```python
from build123d import *

# Parameters (mm, degrees)
SKETCH1_W               = 54
SKETCH1_H               = 32
SKETCH1_R               = 0.95
BOSS_EXTRUDE1_DEPTH     = 2.54
SKETCH3_W               = 3
SKETCH3_H               = 32
BOSS_EXTRUDE2_DEPTH     = 37
SKETCH4_W               = 32
SKETCH4_H               = 3
BOSS_EXTRUDE3_DEPTH     = 47
FILLET1_R               = 2
SKETCH5_R               = 1.425
CUT_EXTRUDE1_DEPTH      = 20
SKETCH8_W               = 32
SKETCH8_H               = 3
BOSS_EXTRUDE4_DEPTH     = 4
SKETCH7_W               = 5
SKETCH7_H               = 26
CUT_EXTRUDE3_DEPTH      = 1
CUT_EXTRUDE3_DEPTH_BACK = 40.54
CHAMFER1_SIZE           = 1.5


with BuildPart() as part:
    # Sketch1 → Boss-Extrude1 (new body)
    with BuildSketch(Plane(origin=(0, 0, 0), x_dir=(1, 0, 0), z_dir=(0, 1, 0))):
        with Locations((1, -10)):
            Rectangle(SKETCH1_W, SKETCH1_H)
        with Locations((-10, 0)):
            Circle(SKETCH1_R, mode=Mode.SUBTRACT)
        with Locations((20, -10)):
            Circle(SKETCH1_R, mode=Mode.SUBTRACT)
        with Locations((-10, -20)):
            Circle(SKETCH1_R, mode=Mode.SUBTRACT)
    extrude(amount=BOSS_EXTRUDE1_DEPTH)

    # Sketch3 → Boss-Extrude2 (add)
    with BuildSketch(Plane(origin=(0, 2.54, 0), x_dir=(1, 0, 0), z_dir=(0, 1, 0))):
        with Locations((26.5, -10)):
            Rectangle(SKETCH3_W, SKETCH3_H)
    extrude(amount=BOSS_EXTRUDE2_DEPTH)

    # Sketch4 → Boss-Extrude3 (add)
    with BuildSketch(Plane.ZY.offset(-25)):
        with Locations((10, 38.04)):
            Rectangle(SKETCH4_W, SKETCH4_H)
    extrude(amount=BOSS_EXTRUDE3_DEPTH)

    # Fillet1
    fillet1_edges = [part.edges().sort_by_distance(p)[0] for p in [
        (28, 0, 10),
        (28, 39.54, 10),
    ]]
    fillet(fillet1_edges, radius=FILLET1_R)

    # Sketch5 → Cut-Extrude1 (cut)
    with BuildSketch(Plane(origin=(0, 39.54, 0), x_dir=(1, 0, 0), z_dir=(0, 1, 0))):
        with Locations((-9.5, 2.5)):
            Circle(SKETCH5_R)
        with Locations((15.5, 2.5)):
            Circle(SKETCH5_R)
        with Locations((15.5, -22.5)):
            Circle(SKETCH5_R)
        with Locations((-9.5, -22.5)):
            Circle(SKETCH5_R)
    extrude(amount=-CUT_EXTRUDE1_DEPTH, mode=Mode.SUBTRACT)

    # Sketch8 → Boss-Extrude4 (add)
    with BuildSketch(Plane.ZY.offset(22)):
        with Locations((10, 38.04)):
            Rectangle(SKETCH8_W, SKETCH8_H)
    extrude(amount=BOSS_EXTRUDE4_DEPTH)

    # Sketch7 → Cut-Extrude3 (cut, two sides)
    with BuildSketch(Plane(origin=(0, 39.54, 0), x_dir=(1, 0, 0), z_dir=(0, 1, 0))) as cut_extrude3_sk:
        with Locations((-21.5, -10)):
            Rectangle(SKETCH7_W, SKETCH7_H)
    extrude(amount=CUT_EXTRUDE3_DEPTH, mode=Mode.SUBTRACT)
    extrude(cut_extrude3_sk.sketch, amount=-CUT_EXTRUDE3_DEPTH_BACK, mode=Mode.SUBTRACT)

    # Chamfer1
    chamfer1_edges = [part.edges().sort_by_distance(p)[0] for p in [
        (25, 2.54, 10),
        (25, 36.54, 10),
    ]]
    chamfer(chamfer1_edges, length=CHAMFER1_SIZE)


solid = part.part
```
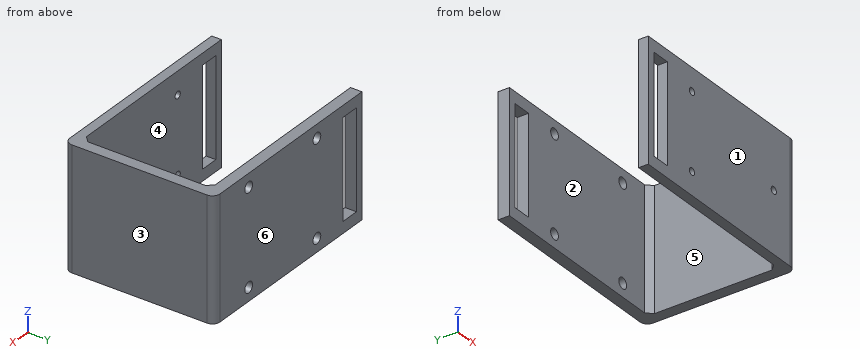
Source: CAD feature listing. Evaluate the final solid. Frame: model axes, mm. Face numbers are marked on the shaded views. A direction names the side the tool comes from. Give positions to 0.01 mm unless a question says otherwise; leave off trailing zeros. Write each loop counter-clockwise with the first axis right and the second up, starting at its lowest first coordinate (ties: lowest second). Pieces come first, ordered by that corner, then holes.
1. Section query D-D (z = 0). Return the cut outline in (x, y), then the cut area to 3 significant figures.
2. First-contact query: pin 1 (5 mm diameter, centred on y = 14.5, z = 1.5, fed in from -X); pin 2 (2.5 mm diameter, centred on x = 15.5, z = -2.5, fed in from +Y); pin 3 (1.1 mm diameter, centred on x = -10, z = 20, fed in from -Y). Flat tips, straight axial feed; report the tip coordinate or a pass-through.
3. Access query for the marked faces 1 and 2. Directions: +Z, -Z, +X, -X, +Y, -Y. A direction counts if a zero-diameter tool reaches every point of the face in a straight line with its end or side. Return the directions, or none.
4. Section query A-A (x = 22). Return the cut outline in (y, z).
5. Section query B-B (x = 15.5). Return the cut outline in (y, z) (3 decimals).
6. Pull-direction query (Y, two-part tool) for the marked faces 3, 4, 5 and 6; classes: +Y half, -Y half, draft (parallel to the pull), parting line (faces both ways), or undercut.
7. Material intervals for line 1 along Z through (x, y) = (-9.5, 37.7) (3 decimals); line 2 along Z through (x, y) = (-10, 1.3); line 3 along Y through (x, z) = (2.5, 3.5), sorted ascending.
8. Section query C-C (z = 17). Return the cut outline in (x, y), then the cut area to 3 significant figures.
Output values:
1. outline: (-26, 0) - (-24, 0) - (-24, 2.54) - (-26, 2.54) - close; (-26, 36.54) - (-24, 36.54) - (-24, 39.54) - (-26, 39.54) - close; (-19, 0) - (-10.95, 0) - (-10.95, 2.54) - (-19, 2.54) - close; (-19, 36.54) - (23.5, 36.54) - (25, 35.04) - (25, 4.04) - (23.5, 2.54) - (-9.05, 2.54) - (-9.05, 0) - (26, 0) arc R2 ccw to (28, 2) - (28, 37.54) arc R2 ccw to (26, 39.54) - (-19, 39.54) - close
1. area: 369 mm2
2. pin 1: stops at x = 25
2. pin 2: stops at y = 2.54
2. pin 3: stops at y = 36.54
3. face 1: +Z, -Z, +X, -X, -Y
3. face 2: +Z, -Z, -X
4. outline: (0, -6) - (2.54, -6) - (2.54, 26) - (0, 26) - close; (36.54, -6) - (39.54, -6) - (39.54, 26) - (36.54, 26) - close
5. outline: (0, -6) - (2.54, -6) - (2.54, 26) - (0, 26) - close; (36.54, -6) - (39.54, -6) - (39.54, -3.925) - (36.54, -3.925) - close; (36.54, -1.075) - (39.54, -1.075) - (39.54, 21.075) - (36.54, 21.075) - close; (36.54, 23.925) - (39.54, 23.925) - (39.54, 26) - (36.54, 26) - close
6. face 3: draft
6. face 4: undercut
6. face 5: undercut
6. face 6: +Y half
7. line 1: z = -6 to -3.925, -1.075 to 21.075, 23.925 to 26
7. line 2: z = -6 to -0.95, 0.95 to 19.05, 20.95 to 26
7. line 3: y = 0 to 2.54, 36.54 to 39.54
8. outline: (-26, 0) - (-24, 0) - (-24, 2.54) - (-26, 2.54) - close; (-26, 36.54) - (-24, 36.54) - (-24, 39.54) - (-26, 39.54) - close; (-19, 0) - (26, 0) arc R2 ccw to (28, 2) - (28, 37.54) arc R2 ccw to (26, 39.54) - (-19, 39.54) - (-19, 36.54) - (23.5, 36.54) - (25, 35.04) - (25, 4.04) - (23.5, 2.54) - (-19, 2.54) - close
8. area: 374 mm2
